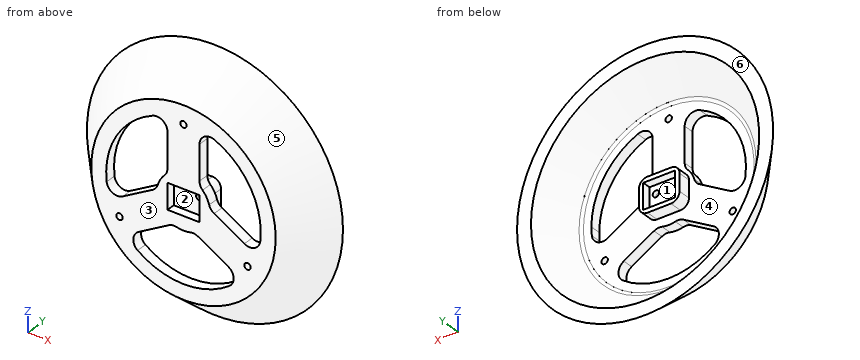
```python
from build123d import *

# Parameters (mm, degrees)
SKETCH1_R                 = 60
BOSS_EXTRUDE1_DEPTH       = 20
BOSS_EXTRUDE1_DRAFT       = -40
SHELL1_T                  = -5
CUT_EXTRUDE2_DEPTH        = 20
SKETCH3_W                 = 15
SKETCH3_H                 = 12
BOSS_EXTRUDE2_DEPTH       = 6
F_3_0MM_DOWEL_HOLE1_D     = 3
FILLET1_R                 = 5
FILLET2_R                 = 2
SKETCH10_W                = 15
SKETCH10_H                = 12
CUT_EXTRUDE3_DEPTH        = 5
SKETCH12_W                = 12
SKETCH12_H                = 3
BOSS_EXTRUDE5_DEPTH       = 7.5
F_3_0MM_DOWEL_HOLE3_D     = 3
F_3_0MM_DOWEL_HOLE3_DEPTH = 15
F_3_0MM_DOWEL_HOLE3_TIP   = 0.901290929


with BuildPart() as part:
    # Sketch1 → Boss-Extrude1 (with draft: the straight prism first)
    with BuildSketch(Plane(origin=(0, 0, 0), x_dir=(1, 0, 0), z_dir=(0, 1, 0))):
        Circle(SKETCH1_R)
    extrude(amount=-BOSS_EXTRUDE1_DEPTH)
    # Boss-Extrude1: the draft: its side faces are tilted about the plane it starts from
    boss_extrude1_sides = [part.faces().sort_by_distance(p)[0] for p in [
        (-60, -10, 0),
    ]]
    draft(boss_extrude1_sides, Plane(origin=(0, 0, 0), x_dir=(1, 0, 0), z_dir=(0, 1, 0)), BOSS_EXTRUDE1_DRAFT)

    # Shell1
    shell1_openings = [part.faces().sort_by_distance(p)[0] for p in [
        (0, 0, 0),
    ]]
    offset(amount=SHELL1_T, openings=shell1_openings, kind=Kind.INTERSECTION)

    # Sketch2 → Cut-Extrude2 (cut)
    with BuildSketch(Plane.XZ.offset(20)):
        with BuildLine():
            ThreePointArc((-7.5, 35.432951589), (-31.365714462, 18.109003688), (-34.435836207, -11.221285266))
            Line((-34.435836207, -11.221285266), (-12.410254038, 1.495190528))
            ThreePointArc((-12.410254038, 1.495190528), (-10.825317547, 6.25), (-7.5, 10))
            Line((-7.5, 10), (-7.5, 35.432951589))
        make_face()
        with BuildLine():
            Line((12.410254038, 1.495190528), (34.435836207, -11.221285266))
            ThreePointArc((34.435836207, -11.221285266), (35.769689879, -5.680963323), (36.218007376, 0))
            ThreePointArc((36.218007376, 0), (28.136978459, 22.804703495), (7.5, 35.432951589))
            Line((7.5, 35.432951589), (7.5, 10))
            ThreePointArc((7.5, 10), (10.825317547, 6.25), (12.410254038, 1.495190528))
        make_face()
        with BuildLine():
            ThreePointArc((-26.935836207, -24.211666323), (0, -36.218007376), (26.935836207, -24.211666323))
            Line((26.935836207, -24.211666323), (4.910254038, -11.495190528))
            ThreePointArc((4.910254038, -11.495190528), (0, -12.5), (-4.910254038, -11.495190528))
            Line((-4.910254038, -11.495190528), (-26.935836207, -24.211666323))
        make_face()
    extrude(amount=-CUT_EXTRUDE2_DEPTH, mode=Mode.SUBTRACT)

    # Sketch3 → Boss-Extrude2 (add)
    with BuildSketch(Plane(origin=(0, -15, 0), x_dir=(1, 0, 0), z_dir=(0, 1, 0))):
        with BuildLine():
            Line((-5.5, -8), (5.5, -8))
            ThreePointArc((5.5, -8), (8.328427125, -6.828427125), (9.5, -4))
            Line((9.5, -4), (9.5, 4))
            ThreePointArc((9.5, 4), (8.328427125, 6.828427125), (5.5, 8))
            Line((5.5, 8), (-5.5, 8))
            ThreePointArc((-5.5, 8), (-8.328427125, 6.828427125), (-9.5, 4))
            Line((-9.5, 4), (-9.5, -4))
            ThreePointArc((-9.5, -4), (-8.328427125, -6.828427125), (-5.5, -8))
        make_face()
        Rectangle(SKETCH3_W, SKETCH3_H, mode=Mode.SUBTRACT)
    extrude(amount=BOSS_EXTRUDE2_DEPTH)

    # Ø3.0mm Dowel Hole1 (through all)
    with Locations(Plane(origin=(0, -15, 0), x_dir=(1, 0, 0), z_dir=(0, 1, 0))):
        with Locations((-29.999119987, 17.32), (29.999119987, 17.32), (0, -34.64)):
            Hole(F_3_0MM_DOWEL_HOLE1_D / 2)

    # Fillet1
    fillet1_edges = [part.edges().sort_by_distance(p)[0] for p in [
        (-26.935836207, -17.5, -24.211666323),
        (-4.910254038, -17.5, -11.495190528),
        (4.910254038, -17.5, -11.495190528),
        (26.935836207, -17.5, -24.211666323),
        (34.435836207, -17.5, -11.221285266),
        (12.410254038, -17.5, 1.495190528),
        (7.5, -17.5, 10),
        (7.5, -17.5, 35.432951589),
        (-7.5, -17.5, 35.432951589),
        (-7.5, -17.5, 10),
        (-12.410254038, -17.5, 1.495190528),
        (-34.435836207, -17.5, -11.221285266),
    ]]
    fillet(fillet1_edges, radius=FILLET1_R)

    # Fillet2
    fillet2_edges = [part.edges().sort_by_distance(p)[0] for p in [
        (-40.886469086, -15, 0),
    ]]
    fillet(fillet2_edges, radius=FILLET2_R)

    # Sketch10 → Cut-Extrude3 (cut)
    with BuildSketch(Plane.XZ.offset(20)):
        Rectangle(SKETCH10_W, SKETCH10_H)
    extrude(amount=-CUT_EXTRUDE3_DEPTH, mode=Mode.SUBTRACT)

    # Sketch12 → Boss-Extrude5 (add, symmetric)
    with BuildSketch(Plane(origin=(0, 0, 0), x_dir=(0, 0, -1), z_dir=(1, 0, 0))):
        with Locations((0, -14.5)):
            Rectangle(SKETCH12_W, SKETCH12_H)
    extrude(amount=BOSS_EXTRUDE5_DEPTH, both=True)

    # Sketch9 → Ø3.0mm Dowel Hole2 (revolve, cut)
    with BuildSketch(Plane(origin=(4.5, -15, 2), x_dir=(0, 0, -1), z_dir=(1, 0, 0))):
        Polygon((0, 0), (0, 15.901290929), (1.5, 15), (1.5, 0), align=None)
    revolve(axis=Axis((4.5, -21.35, 2), (0, 1, 0)), mode=Mode.SUBTRACT)

    # Ø3.0mm Dowel Hole3
    with Locations(Plane(origin=(0, -15, 0), x_dir=(1, 0, 0), z_dir=(0, 1, 0))):
        with Locations((4.5, -2)):
            Hole(F_3_0MM_DOWEL_HOLE3_D / 2, depth=F_3_0MM_DOWEL_HOLE3_DEPTH)
            with Locations((0, 0, -(F_3_0MM_DOWEL_HOLE3_DEPTH + F_3_0MM_DOWEL_HOLE3_TIP / 2))):  # 118° drill point
                Cone(0, F_3_0MM_DOWEL_HOLE3_D / 2, F_3_0MM_DOWEL_HOLE3_TIP, mode=Mode.SUBTRACT)


solid = part.part
```
Work out the finished part from the listing and answer in its coordinate system (mm). Face numbers are marked on the shaded views. A direction names the side the tool comes from. Coordinates: 2 decimals unless noted, no trailing zeros. Loops run counter-clockwise (first coordinate to the right, second up) from the corner with the lowest first, then second, coordinate; pieces in that order, holes last. Notation, with made-up numbers: (20.5, -22) - (54.5, -22) arc R28 ccw to (54.5, 5) - close; hole circle Ø2 at (34.5, 52.5). An arc over 180 degrees is marked (long way). Use a Markdown table: item, result.
Item 1: Find section A-A, the plane x = 0. State how many separate pieces and enclosed holes the cut face has, and give its area (3 significant figures).
Evaluation:
| item | result |
|---|---|
| separate pieces | 3 |
| enclosed holes | 0 |
| area | 516 mm2 |
Item 2: For the marked faces 1, 2 and 3, determine the directions among +Z, -Z, +X, -X, +Y, -Y from which every point of the face is accessible in a straight line to the end or side of a thin tool.
Evaluation:
| item | result |
|---|---|
| face 1 | +Y |
| face 2 | -Y |
| face 3 | +Z, -Z, +X, -X, -Y |
Item 3: Consider probe 1 along Z at (x, y) = (0, -16.5); probe 2 along X at (y, z) = (-17.7, -17.32); probe 3 along Z at (x, y) = (0, -17.75). Determine where each line is inside the solid, lowest interval first. Write a range as from..to.
Evaluation:
| item | result |
|---|---|
| probe 1 | z = -46.15..-36.22, -12.5..-6, 6..33.14, 36.14..46.15 |
| probe 2 | x = -41.69..-31.5, -28.5..-15, 15..28.5, 31.5..41.69 |
| probe 3 | z = -45.11..-36.22, -12.5..-6, 6..33.14, 36.14..45.11 |
Item 4: Given pin 1 Ø6 at (y, z) = (-6.5, 29) entering from -X; pin 2 Ø13 at (x, z) = (0, 2) entering from +Y; pin 3 Ø2.5 at (x, z) = (4.5, 2) entering from +Y; pin 4 Ø8 at (y, z) = (-15.5, 12.5) entering from +X, each flat-ended and moving along its own axis, determine where each tip first touches the part or whether it passes through.
Evaluation:
| item | result |
|---|---|
| pin 1 | stops at x = -49.61 |
| pin 2 | stops at y = -9 |
| pin 3 | passes through |
| pin 4 | stops at x = 48.91 |
Item 5: The mould has two halves that part along Z. Classify the marked faces 4, 5 and 6: +Z half, -Z half, draft (parallel to the pull), parting line (faces both ways), or undercut.
Evaluation:
| item | result |
|---|---|
| face 4 | undercut |
| face 5 | parting line |
| face 6 | draft |
Item 6: Find section C-C, the plane y = -1.75. Determine the outline of the cut face in (x, z).
Evaluation:
| item | result |
|---|---|
| outline | circle Ø117.06 at (0, 0); hole circle Ø104.01 at (0, 0) |
